Source: three-view drawing plus pictorial views. Frame: mm from the lowest corner of the part. A direction names the side the tool comes from. Give positions to 0.01 mm unless a question says otherwise; leave off trailing zeros. Loops run counter-clockwise (first coordinate to the right, second up) from the corner with the lowest first, then second, coordinate; pieces in that order, holes last.
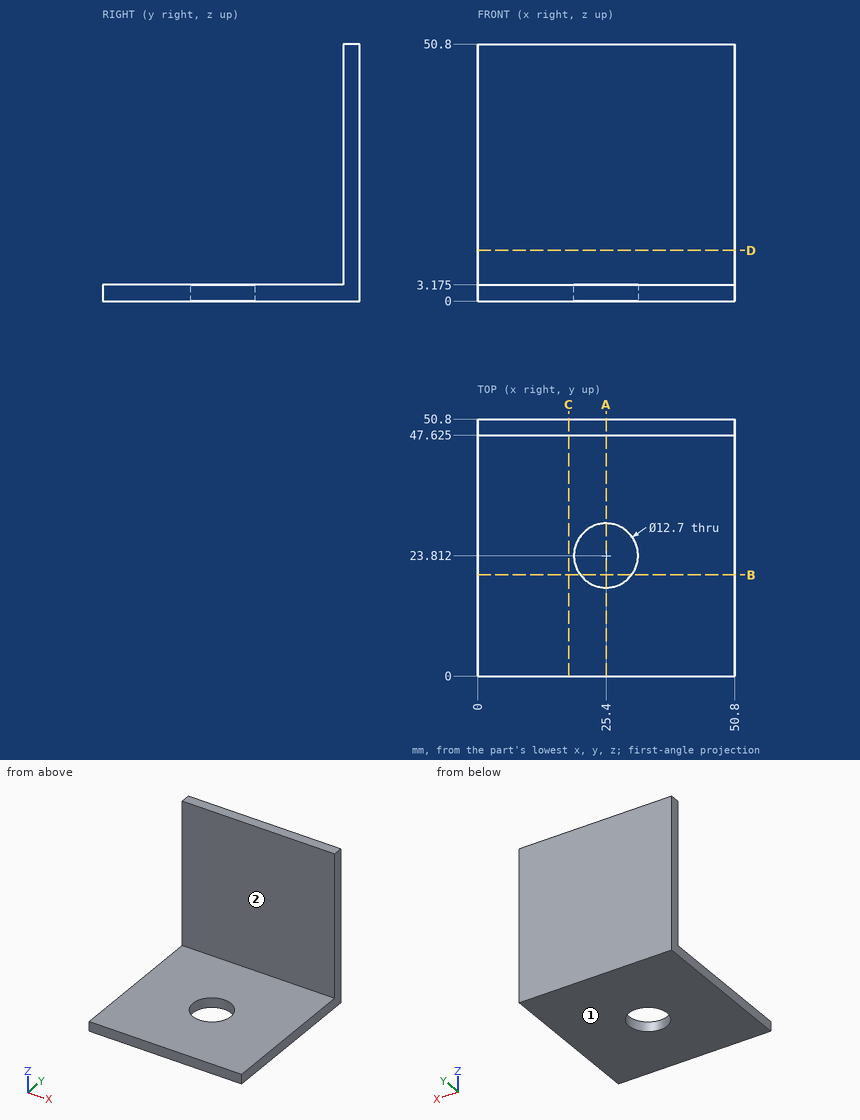
1) Cut plane B-B (y = 20). Return loops of the section in (x, z) (1 decimal).
Checks:
outline: (0, 0) - (20.3, 0) - (20.3, 3.2) - (0, 3.2) - close; (30.5, 0) - (50.8, 0) - (50.8, 3.2) - (30.5, 3.2) - close
2) Contact query for flat-ended pins moving along their axis: P1, Ø12, axis at x = 10, y = 28.5, coming from the +Z side (1 decimal); P2, Ø2, axis at x = 39, z = 34, coming from the -Y side (1 decimal); P3, Ø5, axis at x = 38, y = 38, coming from the -Z side. Output: stop coordinate, or through.
Checks:
P1: stops at z = 3.2
P2: stops at y = 47.6
P3: stops at z = 0
3) Cut plane D-D (z = 10). Return loops of the section in (x, y) (1 decimal).
Checks:
outline: (0, 47.6) - (50.8, 47.6) - (50.8, 50.8) - (0, 50.8) - close
4) Ray query, probe 1 along Z at (x, y) = (45, 36) (1 decimal); probe 2 along Y at (x, z) = (25.4, 1.9); probe 3 along Y at (x, z) = (23.5, 38.5) (1 decimal). Return the intervals inside material, ascending.
Checks:
probe 1: z = 0 to 3.2
probe 2: y = 0 to 17.46, 30.16 to 50.8
probe 3: y = 47.6 to 50.8
5) Cut plane C-C (x = 18). Return loops of the section in (y, z) (1 decimal).
Checks:
outline: (0, 0) - (50.8, 0) - (50.8, 50.8) - (47.6, 50.8) - (47.6, 3.2) - (0, 3.2) - close
6) Reachability of the marked faces 1 and 2 from +Z, -Z, +X, -X, +Y, -Y: full face, straight path, thin tool, end or side. Return the list, or none.
Checks:
face 1: -Z, +X, -X, +Y, -Y
face 2: +Z, +X, -X, -Y
7) Cut plane A-A (x = 25.4). Return loops of the section in (y, z) (1 decimal).
Checks:
outline: (0, 0) - (17.5, 0) - (17.5, 3.2) - (0, 3.2) - close; (30.2, 0) - (50.8, 0) - (50.8, 50.8) - (47.6, 50.8) - (47.6, 3.2) - (30.2, 3.2) - close
